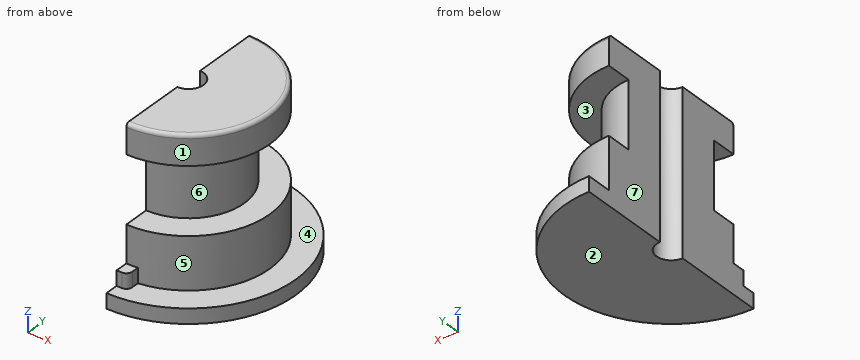
from build123d import *

# Parameters (mm, degrees)
F0_R      = 14.5
F1_DEPTH  = 2
F2_R      = 11
F3_DEPTH  = 20
F4_R      = 2
F5_DEPTH  = 22.001
F6_W      = 3
F6_H      = 3.4
F7_DEPTH  = 2
F8_R      = 0.8
F9_R      = 0.5
F11_W     = 28.85052
F11_H     = 54.144128
F12_DEPTH = 22.001
F14_W     = 3.5
F14_H     = 9


with BuildPart() as f1:
    # F0 (on Top) → F1 (new body)
    with BuildSketch(Plane.XY):
        Circle(F0_R)
    extrude(amount=F1_DEPTH)

    # F2 (on face) → F3 (join)
    with BuildSketch(Plane.XY.offset(2)):
        Circle(F2_R)
    extrude(amount=F3_DEPTH)

    # F4 (on face) → F5 (cut, through all)
    with BuildSketch(Plane(origin=(0, 0, 0), x_dir=(1, 0, 0), z_dir=(0, 0, -1))):
        Circle(F4_R)
    extrude(amount=-F5_DEPTH, mode=Mode.SUBTRACT)

    # F6 (on face) → F7 (join)
    with BuildSketch(Plane.XY.offset(2)):
        with Locations((0, -11)):
            Rectangle(F6_W, F6_H)
    extrude(amount=F7_DEPTH)

    # F8
    f8_edges = [f1.edges().sort_by_distance(p)[0] for p in [
        (-1.5, -12.7, 3),
        (1.5, -12.7, 3),
    ]]
    fillet(f8_edges, radius=F8_R)

    # F9
    f9_edges = [f1.edges().sort_by_distance(p)[0] for p in [
        (-11, 0, 22),
    ]]
    fillet(f9_edges, radius=F9_R)

    # F11 (on Top) → F12 (cut, through all)
    with BuildSketch(Plane.XY):
        with Locations((-14.42526, 2.568883)):
            Rectangle(F11_W, F11_H)
    extrude(amount=F12_DEPTH, mode=Mode.SUBTRACT)

    # F14 (on Front) → F15 (revolve, cut)
    with BuildSketch(Plane.XZ):
        with Locations((9.25, 13.5)):
            Rectangle(F14_W, F14_H)
    revolve(axis=Axis((0, 0, 13.307823), (0, 0, 1)), mode=Mode.SUBTRACT)


solid = f1.part
Here's how the part is built. I have some questions about the finished solid (model axes, mm). Face numbers are marked on the shaded views. A direction names the side the tool comes from. Coordinates: 2 decimals unless noted, no trailing zeros. Loops run counter-clockwise (first coordinate to the right, second up) from the corner with the lowest first, then second, coordinate; pieces in that order, holes last.
1. For the marked faces 5, 6 and 7, which set-ups out of +Z, -Z, +X, -X, +Y, -Y let a thin tool reach every point of the face, with its end or its side?
2. Imagine slicing it at B-B, the plane z = 7.25. Please give me the cut outline in (x, y).
3. Imagine slicing it at A-A, the plane y = 0. Please give me the cut outline in (x, z).
4. Imagine slicing it at C-C, the plane x = 12.75. Please give me the cut outline in (y, z), and give its area (3 significant figures).
5. I need wall thicknesses on L1, parallel to Z at x = 4.25, y = 10.25; L2, parallel to Z at x = 2.5, y = 10.25; L3, parallel to Y at x = 1.75, z = 19.25. Which ranges of each line are inside material? Lowest first, please.
6. For P1, Ø0.8, axis at x = 0.5, z = 2.5, coming from the -Y side; P2, Ø1, axis at x = 8, z = 18.5, coming from the +Y side; P3, Ø12, axis at y = 7, z = 4.5, coming from the +X side, each with a flat end and sliding along its axis, tell me the tip position at first contact or that it passes through.
7. If we mould it in two halves opening along Z, with no side actions, what happens to the marked faces 1, 2, 3 and 4? For each: pulls with the +Z half, pulls with the -Z half, needs draft (parallel to the pull), parting line crosses it, or undercut.
Taken from the geometry:
1. face 5: +Z, +X
1. face 6: +X
1. face 7: +Z, -Z, -X, +Y, -Y
2. outline: (0, -11) arc R11 ccw to (0, 11) - (0, 2) arc R2 cw to (0, -2) - close
3. outline: (2, 0) - (14.5, 0) - (14.5, 2) - (11, 2) - (11, 9) - (7.5, 9) - (7.5, 18) - (11, 18) - (11, 21.5) arc R0.5 ccw to (10.5, 22) - (2, 22) - close
4. outline: (-6.91, 0) - (6.91, 0) - (6.91, 2) - (-6.91, 2) - close
4. area: 27.6 mm2
5. L1: z = 0 to 2
5. L2: z = 0 to 9, 18 to 22
5. L3: y = -10.86 to -0.97, 0.97 to 10.86
6. P1: stops at y = -12.7
6. P2: stops at y = 8.05
6. P3: stops at x = 14.42
7. face 1: needs draft
7. face 2: pulls with the -Z half
7. face 3: undercut
7. face 4: pulls with the +Z half
